Here's how the part is built. I have some questions about the finished solid (model axes, mm). A direction names the side the tool comes from. Round coordinates to 2 decimals unless told otherwise and drop trailing zeros. Write each question's results on one line, items separated by ' | '. Start each with the question number.
```python
from build123d import *

# Parameters (mm, degrees)
F1_DEPTH = 1000


# Not quite as in the source:
# - ends of sketch curves that miss each other by under 0.0002 mm in the source are joined


with BuildPart() as f1:
    # F0 (on Top) → F1 (new body)
    with BuildSketch(Plane.XY):
        with BuildLine():
            Line((23, 9.273618), (23, 14.841657))
            ThreePointArc((23, 14.841657), (23.3912385359, 15.6350103133), (24.2588189596, 15.8075828492))
            Line((24.2588189596, 15.8075828492), (43.426476, 10.671624))
            ThreePointArc((43.426476, 10.671624), (44.5109517857, 10.8873403242), (45, 11.879032))
            Line((45, 11.879032), (45, 39))
            ThreePointArc((45, 39), (43.2426406871, 43.2426406871), (39, 45))
            Line((39, 45), (-39, 45))
            ThreePointArc((-39, 45), (-43.2426406871, 43.2426406871), (-45, 39))
            Line((-45, 39), (-45, -39))
            ThreePointArc((-45, -39), (-43.2426406871, -43.2426406871), (-39, -45))
            Line((-39, -45), (39, -45))
            ThreePointArc((39, -45), (43.2426406871, -43.2426406871), (45, -39))
            Line((45, -39), (45, -11.879032))
            ThreePointArc((45, -11.879032), (44.5109517857, -10.8873403242), (43.4264761923, -10.6716247175))
            Line((43.4264761923, -10.6716247175), (24.258819, -15.807583))
            ThreePointArc((24.258819, -15.807583), (23.3912385359, -15.6350103133), (23, -14.841657))
            Line((23, -14.841657), (23, -9.273618))
            ThreePointArc((23, -9.273618), (23.022474706, -9.062799833), (23.0888885991, -8.8614578186))
            ThreePointArc((23.0888885991, -8.8614578186), (25, 0), (23.0888887851, 8.8614579028))
            ThreePointArc((23.0888887851, 8.8614579028), (23.022474706, 9.062799833), (23, 9.273618))
        make_face()
        with BuildLine():
            Line((15.807583, -24.258819), (10.98686, -42.25))
            Line((10.98686, -42.25), (-10.98686, -42.25))
            Line((-10.98686, -42.25), (-15.807583, -24.258819))
            ThreePointArc((-15.807583, -24.258819), (-15.6350103133, -23.3912385359), (-14.841657, -23))
            Line((-14.841657, -23), (-9.273618, -23))
            ThreePointArc((-9.273618, -23), (-9.062799833, -23.022474706), (-8.8614578186, -23.0888885991))
            ThreePointArc((-8.8614578186, -23.0888885991), (0, -25), (8.8614579028, -23.0888887851))
            ThreePointArc((8.8614579028, -23.0888887851), (9.062799833, -23.022474706), (9.273618, -23))
            Line((9.273618, -23), (14.841657, -23))
            ThreePointArc((14.841657, -23), (15.6350103133, -23.3912385359), (15.807583, -24.258819))
        make_face(mode=Mode.SUBTRACT)
        with BuildLine():
            ThreePointArc((-42.25, -16.440321), (-41.4675229282, -14.8536143733), (-39.7323620808, -14.5084693016))
            Line((-39.7323620808, -14.5084693016), (-24.482362, -18.594694))
            ThreePointArc((-24.482362, -18.594694), (-23.4132933733, -19.3090230718), (-23, -20.526546))
            Line((-23, -20.526546), (-23, -21))
            ThreePointArc((-23, -21), (-22.4142135624, -22.4142135624), (-21, -23))
            Line((-21, -23), (-20.526546, -23))
            ThreePointArc((-20.526546, -23), (-19.3090230718, -23.4132933733), (-18.5946943016, -24.4823620808))
            Line((-18.5946943016, -24.4823620808), (-14.508469, -39.732362))
            ThreePointArc((-14.508469, -39.732362), (-14.8536143733, -41.4675229282), (-16.440321, -42.25))
            Line((-16.440321, -42.25), (-39, -42.25))
            ThreePointArc((-39, -42.25), (-41.2980970389, -41.2980970389), (-42.25, -39))
            Line((-42.25, -39), (-42.25, -16.440321))
        make_face(mode=Mode.SUBTRACT)
        with BuildLine():
            ThreePointArc((16.440321, -42.25), (14.8536143733, -41.4675229282), (14.5084693016, -39.7323620808))
            Line((14.5084693016, -39.7323620808), (18.594694, -24.482362))
            ThreePointArc((18.594694, -24.482362), (19.3090230718, -23.4132933733), (20.526546, -23))
            Line((20.526546, -23), (21, -23))
            ThreePointArc((21, -23), (22.4142135624, -22.4142135624), (23, -21))
            Line((23, -21), (23, -20.526546))
            ThreePointArc((23, -20.526546), (23.4132933733, -19.3090230718), (24.4823620808, -18.5946943016))
            Line((24.4823620808, -18.5946943016), (39.732362, -14.508469))
            ThreePointArc((39.732362, -14.508469), (41.4675229282, -14.8536143733), (42.25, -16.440321))
            Line((42.25, -16.440321), (42.25, -39))
            ThreePointArc((42.25, -39), (41.2980970389, -41.2980970389), (39, -42.25))
            Line((39, -42.25), (16.440321, -42.25))
        make_face(mode=Mode.SUBTRACT)
        with BuildLine():
            Line((-24.258819, -15.807583), (-42.25, -10.98686))
            Line((-42.25, -10.98686), (-42.25, 10.98686))
            Line((-42.25, 10.98686), (-24.258819, 15.807583))
            ThreePointArc((-24.258819, 15.807583), (-23.3912385359, 15.6350103133), (-23, 14.841657))
            Line((-23, 14.841657), (-23, 9.273618))
            ThreePointArc((-23, 9.273618), (-23.022474706, 9.062799833), (-23.0888885991, 8.8614578186))
            ThreePointArc((-23.0888885991, 8.8614578186), (-25, 0), (-23.0888887851, -8.8614579028))
            ThreePointArc((-23.0888887851, -8.8614579028), (-23.022474706, -9.062799833), (-23, -9.273618))
            Line((-23, -9.273618), (-23, -14.841657))
            ThreePointArc((-23, -14.841657), (-23.3912385359, -15.6350103133), (-24.258819, -15.807583))
        make_face(mode=Mode.SUBTRACT)
        with BuildLine():
            ThreePointArc((19.25, 20.25), (19.9571067812, 19.9571067812), (20.25, 19.25))
            Line((20.25, 19.25), (20.25, 7.3951))
            ThreePointArc((20.25, 7.3951), (20.2639867072, 7.2284333074), (20.3055555728, 7.0664288513))
            ThreePointArc((20.3055554887, 7.066428822), (21.5, 0), (20.3055554887, -7.066428822))
            ThreePointArc((20.3055555728, -7.0664288513), (20.2639867072, -7.2284333074), (20.25, -7.3951))
            Line((20.25, -7.3951), (20.25, -19.25))
            ThreePointArc((20.25, -19.25), (19.9571067812, -19.9571067812), (19.25, -20.25))
            Line((19.25, -20.25), (7.3951, -20.25))
            ThreePointArc((7.3951, -20.25), (7.2284333074, -20.2639867072), (7.0664288513, -20.3055555728))
            ThreePointArc((7.066428822, -20.3055554887), (0, -21.5), (-7.066428822, -20.3055554887))
            ThreePointArc((-7.0664288513, -20.3055555728), (-7.2284333074, -20.2639867072), (-7.3951, -20.25))
            Line((-7.3951, -20.25), (-19.25, -20.25))
            ThreePointArc((-19.25, -20.25), (-19.9571067812, -19.9571067812), (-20.25, -19.25))
            Line((-20.25, -19.25), (-20.25, -7.3951))
            ThreePointArc((-20.25, -7.3951), (-20.2639867072, -7.2284333074), (-20.3055555728, -7.0664288513))
            ThreePointArc((-20.3055554887, -7.066428822), (-21.5, 0), (-20.3055554887, 7.066428822))
            ThreePointArc((-20.3055555728, 7.0664288513), (-20.2639867072, 7.2284333074), (-20.25, 7.3951))
            Line((-20.25, 7.3951), (-20.25, 19.25))
            ThreePointArc((-20.25, 19.25), (-19.9571067812, 19.9571067812), (-19.25, 20.25))
            Line((-19.25, 20.25), (-7.3951, 20.25))
            ThreePointArc((-7.3951, 20.25), (-7.2284333074, 20.2639867072), (-7.0664288513, 20.3055555728))
            ThreePointArc((-7.066428822, 20.3055554887), (0, 21.5), (7.066428822, 20.3055554887))
            ThreePointArc((7.0664288513, 20.3055555728), (7.2284333074, 20.2639867072), (7.3951, 20.25))
            Line((7.3951, 20.25), (19.25, 20.25))
        make_face(mode=Mode.SUBTRACT)
        with BuildLine():
            ThreePointArc((-16.440321, 42.25), (-14.8536143733, 41.4675229282), (-14.5084693016, 39.7323620808))
            Line((-14.5084693016, 39.7323620808), (-18.594694, 24.482362))
            ThreePointArc((-18.594694, 24.482362), (-19.3090230718, 23.4132933733), (-20.526546, 23))
            Line((-20.526546, 23), (-21, 23))
            ThreePointArc((-21, 23), (-22.4142135624, 22.4142135624), (-23, 21))
            Line((-23, 21), (-23, 20.526546))
            ThreePointArc((-23, 20.526546), (-23.4132933733, 19.3090230718), (-24.4823620808, 18.5946943016))
            Line((-24.4823620808, 18.5946943016), (-39.732362, 14.508469))
            ThreePointArc((-39.732362, 14.508469), (-41.4675229282, 14.8536143733), (-42.25, 16.440321))
            Line((-42.25, 16.440321), (-42.25, 39))
            ThreePointArc((-42.25, 39), (-41.2980970389, 41.2980970389), (-39, 42.25))
            Line((-39, 42.25), (-16.440321, 42.25))
        make_face(mode=Mode.SUBTRACT)
        with BuildLine():
            ThreePointArc((15.8075828492, 24.2588189596), (15.6350103133, 23.3912385359), (14.841657, 23))
            Line((14.841657, 23), (9.273618, 23))
            ThreePointArc((9.273618, 23), (9.062799833, 23.022474706), (8.8614578186, 23.0888885991))
            ThreePointArc((8.8614578186, 23.0888885991), (0, 25), (-8.8614579028, 23.0888887851))
            ThreePointArc((-8.8614579028, 23.0888887851), (-9.062799833, 23.022474706), (-9.273618, 23))
            Line((-9.273618, 23), (-14.841657, 23))
            ThreePointArc((-14.841657, 23), (-15.6350103133, 23.3912385359), (-15.8075828492, 24.2588189596))
            Line((-15.8075828492, 24.2588189596), (-10.98686, 42.25))
            Line((-10.98686, 42.25), (10.98686, 42.25))
            Line((10.98686, 42.25), (15.8075828492, 24.2588189596))
        make_face(mode=Mode.SUBTRACT)
        with BuildLine():
            ThreePointArc((42.25, 16.440321), (41.4675229282, 14.8536143733), (39.7323620808, 14.5084693016))
            Line((39.7323620808, 14.5084693016), (24.482362, 18.594694))
            ThreePointArc((24.482362, 18.594694), (23.4132933733, 19.3090230718), (23, 20.526546))
            Line((23, 20.526546), (23, 21))
            ThreePointArc((23, 21), (22.4142135624, 22.4142135624), (21, 23))
            Line((21, 23), (20.526546, 23))
            ThreePointArc((20.526546, 23), (19.3090230718, 23.4132933733), (18.5946943016, 24.4823620808))
            Line((18.5946943016, 24.4823620808), (14.508469, 39.732362))
            ThreePointArc((14.508469, 39.732362), (14.8536143733, 41.4675229282), (16.440321, 42.25))
            Line((16.440321, 42.25), (39, 42.25))
            ThreePointArc((39, 42.25), (41.2980970389, 41.2980970389), (42.25, 39))
            Line((42.25, 39), (42.25, 16.440321))
        make_face(mode=Mode.SUBTRACT)
    extrude(amount=F1_DEPTH)


solid = f1.part
```
Item 1: Which directions (+Z, -Z, +X, -X, +Y, -Y) give clear straight access to the entire face, cutting with the end or side of a thin tool? Please do faces 1 (the face through (33.977, -13.204, 493)), 2 (the face through (1, 45, 493)).
Item 2: If we section it at A-A on z = 119: Count the separate pieces of the cut face and the enclosed holes in it, and give its area (3 significant figures).
Item 3: I'm going to push flat-ended pins straight in: pin 1 (8 mm diameter, centred on x = -28, y = -27.5, fed in from +Z); pin 2 (6 mm diameter, centred on y = -10.5, z = 629, fed in from +X); pin 3 (5 mm diameter, centred on y = 4, z = 175.5, fed in from +X). Where does each tip first touch, or does it pass through?
Item 4: If we mould it in two halves opening along X, with no side actions, what happens to faces 3 (the face through (-42.25, -28, 493)), 4 (the face through (45, 25, 493)), 5 (the face through (-1, -45, 493))? For each: released by +X, released by -X, zero draft, split by the parting line, or undercut.
Item 5: I need wall thicknesses on L1, parallel to Y at x = -4.5, z = 519; L2, parallel to X at y = -2, z = 647.5; L3, parallel to Y at x = -10, z = 957. Which ranges of each line are inside material? Lowest first, please.
Numbers:
1) face 1: +Z, -Z | face 2: +Z, -Z, +X, -X, +Y
2) separate pieces: 1 | enclosed holes: 8 | area: 1,860 mm²
3) pin 1: through | pin 2: x = 45 | pin 3: x = 24.95
4) face 3: undercut | face 4: released by +X | face 5: zero draft
5) L1: -45 to -42.25, -24.52 to -21.02, 21.02 to 24.52, 42.25 to 45 | L2: -45 to -42.25, -24.91 to -21.41, 21.41 to 24.91 | L3: -45 to -42.25, -23 to -20.25, 20.25 to 23, 42.25 to 45
